Autodesk Inventor part; units mm, degrees
ref_plane "YZ Plane" through (0, 0, 0) normal (1, 0, 0) x (0, 1, 0)
ref_plane "XZ Plane" through (0, 0, 0) normal (0, 1, 0) x (-1, 0, 0)
ref_plane "XY Plane" through (0, 0, 0) normal (0, 0, 1) x (1, 0, 0)
sketch "Sketch9" plane through (0, 0, 0) normal (0, 1, 0) x (-1, 0, 0)
  line L0 (25, 25) -> (-25, 25)
  line L1 (-25, 25) -> (-25, -25)
  line L2 (-25, -25) -> (25, -25)
  line L3 (25, -25) -> (25, 25)
  line L4 (25, 25) -> (-25, -25) construction
  line L5 (-25, 25) -> (25, -25) construction
  line L6 (-23, 23) -> (23, 23)
  line L7 (23, 23) -> (23, -23)
  line L8 (23, -23) -> (-23, -23)
  line L9 (-23, -23) -> (-23, 23)
  point P0 (0, 0)
  dimension "d172" = 50
  dimension "d173" = 50
  dimension "d174" = 2
extrude "Extrusion3" add sketch "Sketch9" against normal blind 1055
sketch "Sketch10" plane through (0, 0, 0) normal (1, 0, 0) x (0, 1, 0)
  line L0 (0, 25) -> (0, -25) construction
  line L1 (0, 25) -> (-1055, 25) construction
  line L2 (-1055, -25) -> (-1055, 25) construction
  line L3 (0, -25) -> (-1055, -25) construction
  line L4 (-1050, 8.5) -> (-1033, 8.5)
  line L5 (-1033, 8.5) -> (-1033, -8.5)
  line L6 (-1033, -8.5) -> (-1050, -8.5)
  line L7 (-1050, -8.5) -> (-1050, 8.5)
  line L8 (-1050, 8.5) -> (-1033, -8.5) construction
  line L9 (-1033, 8.5) -> (-1050, -8.5) construction
  circle A0 centre (-1041.5, 0) radius 8.5
  line L10 (0, 25) -> (0, -25)
  point P0 (0, 0)
  point P1 (0, 0)
  point P2 (-1055, 0)
  dimension "d177" = 17
  dimension "d178" = 17
  dimension "d191" = 5
extrude "Extrusion4" cut sketch "Sketch10" along normal through all contours A0
pattern_linear "Rectangular Pattern4" count 9 spacing 125 along (0, 1, 0) of "Extrusion4"
properties part number "TKS 3534 FDS WAY tube4" material "Stainless Steel"
Geometry: final body of the model. Coordinates: model frame, mm. A direction names the side the tool comes from. Give positions to 0.01 mm unless a question says otherwise; leave off trailing zeros. Write each loop counter-clockwise with the first axis right and the second up, starting at its lowest first coordinate (ties: lowest second). Pieces come first, ordered by that corner, then holes.
(1) Ray query, line 1 (X direction, y = -299, z = 21.5); line 2 (Z direction, x = 24.15, y = -291.5). Return the intervals inside material, ascending.
(2) Cut plane C-C, the plane y = -41.5. Return loops of the section in (x, z).
(3) Mould query, pull axis X, two halves, no side actions, for faces 4 (the flat face through (0, -520, -23)), 5 (the flat face through (25, -520, 0)), 6 (the flat face through (-23, -520, 0)), 7 (the cylindrical face through (23.986, -47.765, -5.745)). Classes: released by +X, released by -X, zero draft, split by the parting line, or undercut.
(4) First-contact query: P1, Ø19.5, axis at y = -1041.5, z = 0, coming from the +X side; P2, Ø10, axis at y = -791.5, z = 0, coming from the +X side. Flat tips, straight axial feed; report the tip coordinate or a pass-through.
(5) Access query for faces 1 (the flat face through (-25, -520, 0)), 2 (the flat face through (23, -520, 0)), 3 (the cylindrical face through (24, -800, 0)). Directions: +Z, -Z, +X, -X, +Y, -Y. A direction counts if a zero-diameter tool reaches every point of the face in a straight line with its end or side. Return the directions, or none.
(6) Cut plane A-A, the plane x = -11.5. Return loops of the section in (y, z).
(7) Cut plane B-B, the plane y = -863.5. Return loops of the section in (x, z).
Values follow:
1. line 1: x = -25 to -23, 23 to 25
1. line 2: z = -25 to -8.5, 8.5 to 25
2. outline: (-25, -25) - (25, -25) - (25, -8.5) - (23, -8.5) - (23, -23) - (-23, -23) - (-23, 23) - (23, 23) - (23, 8.5) - (25, 8.5) - (25, 25) - (-25, 25) - close
3. face 4: undercut
3. face 5: released by +X
3. face 6: undercut
3. face 7: zero draft
4. P1: stops at x = 25
4. P2: stops at x = -23
5. face 1: +Z, -Z, -X, +Y, -Y
5. face 2: +Y, -Y
5. face 3: +X
6. outline: (-1055, -25) - (0, -25) - (0, -23) - (-1055, -23) - close; (-1055, 23) - (0, 23) - (0, 25) - (-1055, 25) - close
7. outline: (-25, -25) - (25, -25) - (25, 25) - (-25, 25) - close; hole (-23, -23) - (23, -23) - (23, 23) - (-23, 23) - close
